from build123d import *

# Parameters (mm, degrees)
SKETCH2_W           = 73.039929049
SKETCH2_H           = 6.35
BOSS_EXTRUDE1_DEPTH = 95.25
SKETCH3_R           = 1.75
CUT_EXTRUDE1_DEPTH  = 7.35
CUT_EXTRUDE2_DEPTH  = 7.35
FILLET1_R           = 5.08
SKETCH8_W           = 6.990804807
SKETCH8_H           = 19.05
SKETCH8_H_2         = 50.8
CUT_EXTRUDE3_DEPTH  = 7.35
SKETCH9_W           = 12.7
SKETCH9_H           = 6.35
CUT_EXTRUDE4_DEPTH  = 7.35
LPATTERN1_COUNT     = 8
LPATTERN1_PITCH     = 25.4
SKETCH10_W          = 6.379369351
SKETCH10_H          = 15.875
SKETCH10_H_2        = 12.7
CUT_EXTRUDE5_DEPTH  = 7.35


with BuildPart() as part:
    # Sketch2 → Boss-Extrude1 (new body)
    with BuildSketch(Plane.XY):
        with Locations((40.188577261, 34.925)):
            Rectangle(SKETCH2_W, SKETCH2_H)
    extrude(amount=BOSS_EXTRUDE1_DEPTH)

    # Sketch3 → Cut-Extrude1 (cut, through all)
    with BuildSketch(Plane(origin=(0, 38.1, 0), x_dir=(1, 0, 0), z_dir=(0, 1, 0))):
        with Locations((17.308541785, -26.75)):
            Circle(SKETCH3_R)
        with Locations((17.308541785, -36.75)):
            Circle(SKETCH3_R)
        with Locations((65.308541785, -36.75)):
            Circle(SKETCH3_R)
        with Locations((65.308541785, -26.75)):
            Circle(SKETCH3_R)
        Polygon((64.168541785, -29.21), (64.168541785, -34.29), (61.628541785, -36.83), (61.628541785, -41.91), (20.988541785, -41.91), (20.988541785, -21.59), (61.628541785, -21.59), (61.628541785, -26.67), align=None)
    extrude(amount=-CUT_EXTRUDE1_DEPTH, mode=Mode.SUBTRACT)

    # Sketch6 → Cut-Extrude2 (cut, through all)
    with BuildSketch(Plane(origin=(0, 38.1, 0), x_dir=(1, 0, 0), z_dir=(0, 1, 0))):
        with BuildLine():
            Line((57.56896905, -48.26), (70.388541785, -48.26))
            Line((70.388541785, -48.26), (70.388541785, -12.664576304))
            ThreePointArc((70.388541785, -12.664576304), (73.417894551, -9.376528703), (76.708541785, -6.35))
            Line((76.708541785, -6.35), (76.708541785, -88.9))
            ThreePointArc((76.708541785, -88.9), (62.718427414, -70.661771391), (57.56896905, -48.26))
        make_face()
    extrude(amount=-CUT_EXTRUDE2_DEPTH, mode=Mode.SUBTRACT)

    # Fillet1
    fillet1_edges = [part.edges().sort_by_distance(p)[0] for p in [
        (57.56896905, 34.925, 48.26),
        (70.388541785, 34.925, 48.26),
        (70.388541785, 34.925, 12.664576304),
    ]]
    fillet(fillet1_edges, radius=FILLET1_R)

    # Sketch8 → Cut-Extrude3 (cut, through all)
    with BuildSketch(Plane(origin=(0, 38.1, 0), x_dir=(1, 0, 0), z_dir=(0, 1, 0))):
        with Locations((45.079952064, -9.525)):
            Rectangle(SKETCH8_W, SKETCH8_H)
        with Locations((45.079952064, -69.85)):
            Rectangle(SKETCH8_W, SKETCH8_H_2)
    extrude(amount=-CUT_EXTRUDE3_DEPTH, mode=Mode.SUBTRACT)

    # Sketch9 → Cut-Extrude4 (cut, through all)
    with BuildSketch(Plane(origin=(0, 38.1, 0), x_dir=(1, 0, 0), z_dir=(0, 1, 0))):
        with Locations((57.658541785, -3.175)):
            Rectangle(SKETCH9_W, SKETCH9_H)
        with Locations((57.658541785, -92.075)):
            Rectangle(SKETCH9_W, SKETCH9_H)
    cut_extrude4 = extrude(amount=-CUT_EXTRUDE4_DEPTH, mode=Mode.SUBTRACT)

    # LPattern1: Cut-Extrude4 ×8
    with Locations(*[(-i * LPATTERN1_PITCH, 0, 0) for i in range(1, LPATTERN1_COUNT)]):
        add(cut_extrude4, mode=Mode.SUBTRACT)

    # Sketch10 → Cut-Extrude5 (cut, through all)
    with BuildSketch(Plane(origin=(0, 38.1, 0), x_dir=(1, 0, 0), z_dir=(0, 1, 0))):
        with Locations((6.858297412, -7.9375)):
            Rectangle(SKETCH10_W, SKETCH10_H)
        with Locations((6.858297412, -87.3125)):
            Rectangle(SKETCH10_W, SKETCH10_H)
        with Locations((6.858297412, -60.325)):
            Rectangle(SKETCH10_W, SKETCH10_H_2)
        with Locations((6.858297412, -34.925)):
            Rectangle(SKETCH10_W, SKETCH10_H_2)
    extrude(amount=-CUT_EXTRUDE5_DEPTH, mode=Mode.SUBTRACT)


solid = part.part
For this review, take the finished solid that the model builds, in its own axes (mm). A direction names the side the tool comes from. Coordinates: 2 decimals unless noted, no trailing zeros. Loops run counter-clockwise (first coordinate to the right, second up) from the corner with the lowest first, then second, coordinate; pieces in that order, holes last. Notation, with made-up numbers: (15, 54.25) - (55, 54.25) arc R36 cw to (55, 91.25) - close; hole circle Ø6 at (53, 38). An arc over 180 degrees is marked (long way). Return JSON: item names as keys, results as strings.
Item 1: For line 1 (X direction, y = 35.75, z = 26.5); line 2 (X direction, y = 38, z = 37); line 3 (Z direction, x = 29, y = 34.5), list the stretches that pass through material, from the lowest coordinate up.
Determined:
{"line 1": "x = 3.67 to 15.58, 19.04 to 20.99, 61.63 to 63.58, 67.04 to 70.39", "line 2": "x = 10.05 to 15.58, 19.04 to 20.99, 61.63 to 63.58, 67.04 to 70.39", "line 3": "z = 6.35 to 21.59, 41.91 to 88.9"}
Item 2: Take a section at B-B (z = 60). Give the boundary of the cut face in (x, y), then the cut area to 3 significant figures.
Determined:
{"outline": "(10.05, 31.75) - (41.58, 31.75) - (41.58, 38.1) - (10.05, 38.1) - close; (48.58, 31.75) - (59, 31.75) - (59, 38.1) - (48.58, 38.1) - close", "area": "266 mm2"}
Item 3: Take a section at A-A (x = 36.5). Give the boundary of the cut face in (y, z).
Determined:
{"outline": "(31.75, 6.35) - (38.1, 6.35) - (38.1, 21.59) - (31.75, 21.59) - close; (31.75, 41.91) - (38.1, 41.91) - (38.1, 88.9) - (31.75, 88.9) - close"}
Item 4: Take a section at C-C (y = 35.75). State how many separate pieces and enclosed holes the cut face has, then the cut area to 3 significant figures.
Determined:
{"separate pieces": "1", "enclosed holes": "5", "area": "4,080 mm2"}
Item 5: Insertion check: pin 1 (1.5 mm diameter, centred on x = 17.5, z = 35.5, fed in from +Y); pin 2 (1.9 mm diameter, centred on y = 36.5, z = 59, fed in from -X); pin 3 (1 mm diameter, centred on x = 59.5, y = 33, fed in from -Z); pin 4 (3 mm diameter, centred on x = 6.5, y = 36, fed in from -Z) (3 decimals). Each pin has a flat end and moves straight along its axis. Give the tip position at first contact, or say it passes through.
Determined:
{"pin 1": "stops at y = 38.1", "pin 2": "stops at x = 10.05", "pin 3": "stops at z = 6.35", "pin 4": "stops at z = 15.875"}
Item 6: For faces 5 (the flat face through (61.629, 35, 24)), 6 (the flat face through (64.009, 35, 92)), 7 (the flat face through (45, 35, 19.05)), 8 (the flat face through (7, 35, 41.275)), list the 3-axis set-ups (+Z, -Z, +X, -X, +Y, -Y) from which the entire face can be reached by the end or side of a thin tool; tool diameter is ignored.
Determined:
{"face 5": "+Y, -Y", "face 6": "+Z, +Y, -Y", "face 7": "-Z, +Y, -Y", "face 8": "-X, +Y, -Y"}
Item 7: Mouldability with a two-part tool opening along X and no side actions: class faces 1 (the flat face through (25.909, 35, 92)), 2 (the flat face through (3.669, 35, 48)), 3 (the flat face through (70.389, 35, 29)), 4 (the flat face through (7, 35, 15.875)) as pulls with the +X half, pulls with the -X half, needs draft (parallel to the pull), parting line crosses it, or undercut.
Determined:
{"face 1": "undercut", "face 2": "pulls with the -X half", "face 3": "pulls with the +X half", "face 4": "needs draft"}
